Input: part model. Units: mm. Frame: model coordinates. A direction names the side the tool comes from. Coordinates: 2 decimals unless noted, no trailing zeros. Write each loop counter-clockwise with the first axis right and the second up, starting at its lowest first coordinate (ties: lowest second). Pieces come first, ordered by that corner, then holes. Notation, with made-up numbers: (-27.75, -37.75) - (-22.75, -37.75) arc R11 ccw to (-22.75, -33.75) - close; hole circle Ø6 at (-26, 39). An arc over 180 degrees is marked (long way). Use a Markdown table: item, result. Add a question column.
Q1. Section query B-B (x = 0). Return the cut outline in (y, z).
Q2. Section query C-C (y = -397). Return the cut outline in (x, z), then the cut area to 3 significant figures.
Q3. Mould query, pull axis Z, two halves, no side actions, for faces 1 (the face through (24, -467.97, -24)), 2 (the face through (-57.095, -185.994, 2.513)), 3 (the face through (0, -382.27, 0)). Classes: released by +Z, released by -Z, zero draft, split by the parting line, or undercut.
Q4. Pin query (flat end, axial travel): P1, Ø6, axis at y = -159, z = 1, coming from the +X side; P2, Ø6, axis at x = -27.5, y = -264.5, coming from the -Z side; P3, Ø10, axis at x = 9.5, y = -290, coming from the +Z side. Return the tip coordinate at first contact, or that it passes through.
Q5. Material intervals for probe 1 along Z at (x, y) = (0, -439); probe 2 along Y at (x, z) = (74.5, 10.5); probe 3 along Z at (x, y) = (52, -214.5), sorted ascending. Write a range as from..to.
Q6. Section query D-D (y = -98). Return the cut outline in (x, z), then the cut area to 3 significant figures.
Q7. Section query A-A (z = 0). Return the cut outline in (x, y), then the cut area to 3 significant figures.
Q8. Set-up query: faces 4 (the face through (90.617, 23.664, 28.537)), 5 (the face through (41, 0, -41)). Return all of +Z, -Z, +X, -X, +Y, -Y with unobstructed straight access to the full face (end or side cutting, diameter ignored); none if empty.
from build123d import *

# Parameters (mm, degrees)
F0_R        = 57.15
F1_DEPTH    = 382.27
F2_R        = 95.004000019
F3_DEPTH    = 53
F4_R        = 5
F5_R        = 55
F5_R_2      = 30
F6_DEPTH    = 85.7
F7_S5_R     = 55
F7_T6_DEPTH = 82


# Not quite as in the source:
# - a fillet or chamfer that OpenCascade refuses, or shapes differently, is made with other operations: its cross-section is extruded or revolved along the edge and cut away or added


with BuildPart() as f1:
    # F0 (on Front) → F1 (new body)
    with BuildSketch(Plane.XZ):
        Circle(F0_R)
    extrude(amount=F1_DEPTH)

    # F2 (on Front) → F3 (join)
    with BuildSketch(Plane.XZ):
        Circle(F2_R)
    extrude(amount=-F3_DEPTH)

    # F4
    f4_edges = [f1.edges().sort_by_distance(p)[0] for p in [
        (-95.004, 53, 0),
    ]]
    fillet(f4_edges, radius=F4_R)

    # F5 (on face) → F6 (join)
    with BuildSketch(Plane.XZ.offset(382.27)):
        Circle(F5_R)
        Circle(F5_R_2, mode=Mode.SUBTRACT)
    extrude(amount=F6_DEPTH)

    # F7: chamfer of 5 on 1 edges, made by hand


with BuildPart() as f7_tool2:
    # F7_s3 → F7_t4 (revolve)
    with BuildSketch(Plane.XY):
        Polygon((57.15, -377.27), (52.15, -382.27), (57.15, -382.27), align=None)
    revolve(axis=Axis((0, -382.27, 0), (0, -1, 0)))

    # F7_s5 → F7_t6 (cut, symmetric)
    with BuildSketch(Plane.XZ.offset(379.8)):
        Circle(F7_S5_R)
    extrude(amount=F7_T6_DEPTH, both=True, mode=Mode.SUBTRACT)


with BuildPart() as f1_1:
    add(f1.part)

    # F7_t1: cut F7_tool2
    add(f7_tool2.part, mode=Mode.SUBTRACT)


solid = f1_1.part
Values follow:
| question | item | result |
|---|---|---|
| 1 | outline | (-467.97, -55) - (-379.42, -55) - (-377.27, -57.15) - (0, -57.15) - (0, -95) - (48, -95) arc R5 ccw to (53, -90) - (53, 90) arc R5 ccw to (48, 95) - (0, 95) - (0, 57.15) - (-377.27, 57.15) - (-379.42, 55) - (-467.97, 55) - (-467.97, 30) - (-382.27, 30) - (-382.27, -30) - (-467.97, -30) - close |
| 2 | outline | circle Ø110 at (0, 0); hole circle Ø60 at (0, 0) |
| 2 | area | 6,680 mm2 |
| 3 | face 1 | zero draft |
| 3 | face 2 | split by the parting line |
| 3 | face 3 | undercut |
| 4 | P1 | x = 57.15 |
| 4 | P2 | z = -51.63 |
| 4 | P3 | z = 56.97 |
| 5 | probe 1 | -55..-30, 30..55 |
| 5 | probe 2 | 0..53 |
| 5 | probe 3 | -23.71..23.71 |
| 6 | outline | circle Ø114.3 at (0, 0) |
| 6 | area | 10,300 mm2 |
| 7 | outline | (-95, 0) - (-57.15, 0) - (-57.15, -377.27) - (-55, -379.42) - (-55, -467.97) - (-30, -467.97) - (-30, -382.27) - (30, -382.27) - (30, -467.97) - (55, -467.97) - (55, -379.42) - (57.15, -377.27) - (57.15, 0) - (95, 0) - (95, 48) arc R5 ccw to (90, 53) - (-90, 53) arc R5 ccw to (-95, 48) - close |
| 7 | area | 58,000 mm2 |
| 8 | face 4 | +Y, -Y |
| 8 | face 5 | -Y |
